Geometry check sheet. Reference: the model listing, model coordinates, mm. Round coordinates to 2 decimals unless told otherwise and drop trailing zeros. Write each loop counter-clockwise with the first axis right and the second up, starting at its lowest first coordinate (ties: lowest second). Pieces come first, ordered by that corner, then holes. Notation, with made-up numbers: (38.25, -0.75) -> (92.25, -0.75) arc R15 ccw to (92.25, 10.25) -> close; hole circle Ø3 at (-37.5, 88). An arc over 180 degrees is marked (long way). One line per question, with ' | ' between items.
```python
from build123d import *

# Parameters (mm, degrees)
SKETCH1_W           = 200
SKETCH1_H           = 60
BOSS_EXTRUDE1_DEPTH = 6
SKETCH2_W           = 20
SKETCH2_H           = 6
CUT_EXTRUDE1_DEPTH  = 10
LPATTERN1_COUNT     = 5
LPATTERN1_PITCH     = 40
SKETCH3_W           = 6
SKETCH3_H           = 20
CUT_EXTRUDE2_DEPTH  = 10
SKETCH4_W           = 6
SKETCH4_H           = 20
CUT_EXTRUDE3_DEPTH  = 10
SKETCH6_W           = 6
SKETCH6_H           = 14
CUT_EXTRUDE4_DEPTH  = 10
SKETCH7_W           = 6
SKETCH7_H           = 14
CUT_EXTRUDE5_DEPTH  = 10


with BuildPart() as part:
    # Sketch1 → Boss-Extrude1 (new body)
    with BuildSketch(Plane.XY):
        with Locations((-120.231213873, 116.098265896)):
            Rectangle(SKETCH1_W, SKETCH1_H)
    extrude(amount=BOSS_EXTRUDE1_DEPTH)

    # Sketch2 → Cut-Extrude1 (cut)
    with BuildSketch(Plane(origin=(0, 0, 0), x_dir=(-1, 0, 0), z_dir=(0, 0, -1))):
        with Locations((30.231213873, 89.098265896)):
            Rectangle(SKETCH2_W, SKETCH2_H)
    cut_extrude1 = extrude(amount=-CUT_EXTRUDE1_DEPTH, mode=Mode.SUBTRACT)

    # LPattern1: Cut-Extrude1 ×5
    with Locations(*[(-i * LPATTERN1_PITCH, 0, 0) for i in range(1, LPATTERN1_COUNT)]):
        add(cut_extrude1, mode=Mode.SUBTRACT)

    # Sketch3 → Cut-Extrude2 (cut)
    with BuildSketch(Plane(origin=(0, 0, 0), x_dir=(-1, 0, 0), z_dir=(0, 0, -1))):
        with Locations((217.231213873, 136.098265896)):
            Rectangle(SKETCH3_W, SKETCH3_H)
    extrude(amount=-CUT_EXTRUDE2_DEPTH, mode=Mode.SUBTRACT)

    # Sketch4 → Cut-Extrude3 (cut)
    with BuildSketch(Plane(origin=(0, 0, 0), x_dir=(-1, 0, 0), z_dir=(0, 0, -1))):
        with Locations((23.231213873, 136.098265896)):
            Rectangle(SKETCH4_W, SKETCH4_H)
    extrude(amount=-CUT_EXTRUDE3_DEPTH, mode=Mode.SUBTRACT)

    # Sketch6 → Cut-Extrude4 (cut)
    with BuildSketch(Plane(origin=(0, 0, 0), x_dir=(-1, 0, 0), z_dir=(0, 0, -1))):
        with Locations((217.231213873, 99.098265896)):
            Rectangle(SKETCH6_W, SKETCH6_H)
    extrude(amount=-CUT_EXTRUDE4_DEPTH, mode=Mode.SUBTRACT)

    # Sketch7 → Cut-Extrude5 (cut)
    with BuildSketch(Plane(origin=(0, 0, 0), x_dir=(-1, 0, 0), z_dir=(0, 0, -1))):
        with Locations((23.231213873, 99.098265896)):
            Rectangle(SKETCH7_W, SKETCH7_H)
    extrude(amount=-CUT_EXTRUDE5_DEPTH, mode=Mode.SUBTRACT)


solid = part.part
```
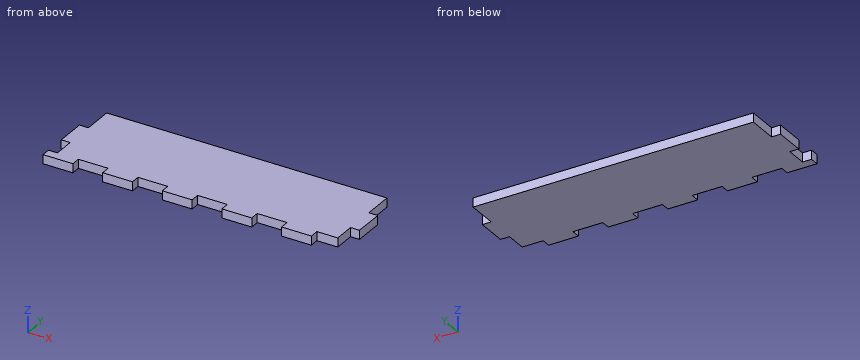
(1) Material ranges on line 1 (X direction, y = 131, z = 5.6); line 2 (Y direction, x = -30.5, z = 2.25), recorded low to high.
Resolved:
line 1: x = -214.23 to -26.23 | line 2: y = 92.1 to 146.1
(2) Go/stop test with flat-tipped pins: pin 1 (3 mm diameter, centred on x = -217, z = 2, fed in from +Y); pin 2 (1.8 mm diameter, centred on x = -111.5, z = 3, fed in from -Y); pin 3 (3 mm diameter, centred on x = -24.5, z = 3.5, fed in from -Y). Record where each tip stops, or that it passes through.
Resolved:
pin 1: stops at y = 126.1 | pin 2: stops at y = 92.1 | pin 3: stops at y = 106.1
(3) Sectioned sample at B-B on x = -144. Record the cut outline in (y, z).
Resolved:
outline: (92.1, 0) -> (146.1, 0) -> (146.1, 6) -> (92.1, 6) -> close
(4) Sectioned sample at C-C on y = 136.5. Record the cut outline in (x, z).
Resolved:
outline: (-214.23, 0) -> (-26.23, 0) -> (-26.23, 6) -> (-214.23, 6) -> close
